CAD build for the part. Positions are in the model's coordinates, mm. Face numbers are marked on the shaded views. A direction names the side the tool comes from. Coordinates: 2 decimals unless noted, no trailing zeros. Order: outer loops, then holes, each group sorted by start corner. A loop starts at its lowest first (then second) coordinate and runs counter-clockwise, first axis right, second up. Notation, with made-up numbers: (2.25, 30) - (21.25, 30) arc R7 ccw to (21.25, 35) - close; hole circle Ø9 at (38.25, -20). An arc over 180 degrees is marked (long way). Return JSON: item names as keys, results as strings.
Autodesk Inventor part; units mm, degrees
ref_plane "XZ Plane" through (0, 0, 0) normal (0, 1, 0) x (-1, 0, 0)
ref_plane "XY Plane" through (0, 0, 0) normal (0, 0, 1) x (1, 0, 0)
sketch "草图1" plane through (0, 0, 0) normal (0, 1, 0) x (-1, 0, 0)
  line L0 (234.2186, 0) -> (-293.6058, 0)
  line L1 (7.25, 23.5) -> (-7.25, 23.5)
  line L2 (-7.25, -23.5) -> (7.25, -23.5)
  line L3 (7.25, -23.5) -> (7.25, 23.5)
  line L4 (7.25, 23.5) -> (-7.25, -23.5) construction
  line L5 (-7.25, 23.5) -> (7.25, -23.5) construction
  line L6 (-7.25, 15.5) -> (-0.75, 15.5)
  line L7 (-0.75, 15.5) -> (-0.75, -15.5)
  line L8 (-0.75, -15.5) -> (-7.25, -15.5)
  line L9 (-13.75, 15.5) -> (-0.75, -15.5) construction
  line L10 (-0.75, 15.5) -> (-13.75, -15.5) construction
  line L11 (-7.25, 23.5) -> (-7.25, 15.5)
  line L12 (-7.25, -15.5) -> (-7.25, -23.5)
  point P0 (0, 0)
  point P1 (-7.25, 0)
  dimension "d0" = 14.5
  dimension "d1" = 47
  dimension "d2" = 13
sketch "草图2" plane through (0, 0, 0) normal (0, 1, 0) x (-1, 0, 0)
  point P0 (0, 0)
sketch "草图3" plane through (0, 0, 0) normal (0, 0, 1) x (1, 0, 0)
  line L0 (0, 0) -> (0, 27)
  arc A0 (32.5, 27) -> (0, 27) centre (16.25, 27) ccw
  line L1 (32.5, 27) -> (32.5, 0)
  dimension "d4" = 27
  dimension "d5" = 32.5
sweep "扫掠1" add profiles "草图1" path "草图3"
sketch "草图4" plane through (7.25, 0, -23.5) normal (0, 0, -1) x (-1, 0, 0)
  line L0 (-18, 27) -> (-18, 0)
  arc A0 (0, 27) -> (-18, 27) centre (-9, 27) ccw
  line L1 (0, 0) -> (0, 27)
  arc A1 (-18, 27) -> (0, 27) centre (-9, 27) ccw
  line L2 (-18, 9) -> (0, 9)
  line L3 (-18, 9) -> (-18, 27)
  line L4 (0, 9) -> (0, 27)
  point P0 (7.25, 0)
  dimension "d7" = 18
extrude "拉伸1" add sketch "草图4" against normal blind 8 contours A1 L1 L2 L0
sketch "草图5" plane through (-7.25, 0, 23.5) normal (0, -1, 0) x (1, 0, 0)
  line L0 (0, 0) -> (14.5, 0)
  line L1 (0, -47) -> (0, 0)
  line L2 (14.5, -47) -> (0, -47)
  line L3 (14.5, -39) -> (14.5, -47)
  line L4 (8, -39) -> (14.5, -39)
  line L5 (8, -8) -> (8, -39)
  line L6 (14.5, -8) -> (8, -8)
  line L7 (14.5, 0) -> (14.5, -8)
  point P0 (7.25, -23.5)
sketch "草图6" plane through (25.25, 0, 23.5) normal (0, -1, 0) x (1, 0, 0)
  line L0 (14.5, 0) -> (0, 0)
  line L1 (0, 0) -> (0, -8)
  line L2 (0, -8) -> (6.5, -8)
  line L3 (6.5, -8) -> (6.5, -39)
  line L4 (6.5, -39) -> (0, -39)
  line L5 (0, -39) -> (0, -47)
  line L6 (0, -47) -> (14.5, -47)
  line L7 (14.5, -47) -> (14.5, 0)
  point P0 (-25.25, -23.5)
sketch "草图7" plane through (-7.25, 0, 23.5) normal (0, -1, 0) x (1, 0, 0)
  line L0 (0, 0) -> (14.5, 0)
  line L1 (0, -47) -> (0, 0)
  line L2 (14.5, -47) -> (0, -47)
  line L3 (14.5, -39) -> (14.5, -47)
  line L4 (8, -39) -> (14.5, -39)
  line L5 (8, -8) -> (8, -39)
  line L6 (14.5, -8) -> (8, -8)
  line L7 (14.5, 0) -> (14.5, -8)
  point P0 (7.25, -23.5)
  dimension "d10" = 6.5
sketch "草图8" plane through (-7.25, 0, 23.5) normal (0, -1, 0) x (1, 0, 0)
  line L0 (8, -8) -> (8, -39)
  circle A0 centre (23.5, -23.5) radius 9
  point P0 (7.25, -23.5)
  dimension "d11" = 18
  dimension "d12" = 15.5
extrude "拉伸2" cut sketch "草图8" against normal blind 232
sketch "草图9" plane through (-7.25, 0, -23.5) normal (-1, 0, 0) x (0, 0, 1)
  line L0 (42.5, 0) -> (4.5, 0)
  line L1 (4.5, 0) -> (4.5, 20)
  line L2 (4.5, 20) -> (42.5, 20)
  line L3 (42.5, 20) -> (42.5, 0)
  line L4 (42.5, 0) -> (4.5, 20) construction
  line L5 (4.5, 0) -> (42.5, 20) construction
  line L6 (47, 0) -> (39, 0)
  point P0 (23.5, 0)
  point P1 (23.5, 10)
  point P2 (43, 0)
  dimension "d15" = 38
  dimension "d16" = 20
ref_plane "工作平面1" through (-3.625, 0, 0) normal (1, 0, 0) x (0, 1, 0)
ref_plane "工作平面2" through (-32.25, 0, -23.5) normal (-1, 0, 0) x (0, 0, 1)
sketch "草图10" plane through (-32.25, 0, -23.5) normal (-1, 0, 0) x (0, 0, 1)
  line L0 (12, 0) -> (35, 0)
  line L1 (35, 0) -> (35, 10)
  line L2 (35, 10) -> (12, 10)
  line L3 (12, 10) -> (12, 0)
  line L4 (12, 0) -> (35, 10) construction
  line L5 (35, 0) -> (12, 10) construction
  point P0 (23.5, 0)
  point P1 (23.5, 5)
  point P2 (39, 0)
  dimension "d18" = 23
  dimension "d19" = 10
loft "放样1" add profiles "草图10", "草图9"
sketch "草图11" plane through (-32.25, 0, 11.5) normal (-1, 0, 0) x (0, 0, 1)
  line L0 (-23, 0) -> (0, 0)
  line L1 (0, 0) -> (0, 10)
  line L2 (0, 10) -> (-23, 10)
  line L3 (-23, 10) -> (-23, 0)
  point P0 (-11.5, 0)
sketch "草图12" plane through (-7.25, 0, 23.5) normal (0, -1, 0) x (1, 0, 0)
  line L0 (-25, -35) -> (-25, -12)
  line L1 (-15, -29.113) -> (-25, -29.113)
  line L2 (-25, -29.113) -> (-25, -17.887)
  line L3 (-25, -17.887) -> (-15, -17.887)
  line L4 (-15, -17.887) -> (-15, -29.113)
  line L5 (-15, -29.113) -> (-25, -17.887) construction
  line L6 (-25, -29.113) -> (-15, -17.887) construction
  point P0 (7.25, -23.5)
  point P1 (-20, -23.5)
  point P2 (-25, -23.5)
  dimension "d24" = 10
extrude "拉伸3" cut sketch "草图12" against normal blind 232
equation "\"折弯半径\" = 厚度"
equation "\"折弯释压宽度\" = 厚度"
equation "\"折弯释压深度\" = 0.5 * 厚度"
equation "\"拐角释压尺寸\" = 4 * 厚度"
equation "\"最小余量\" = 2 * 厚度"
equation "\"过渡半径\" = 折弯半径"
equation "\"Jacobi半径尺寸\" = 厚度"
equation "\"间隙大小\" = 厚度"
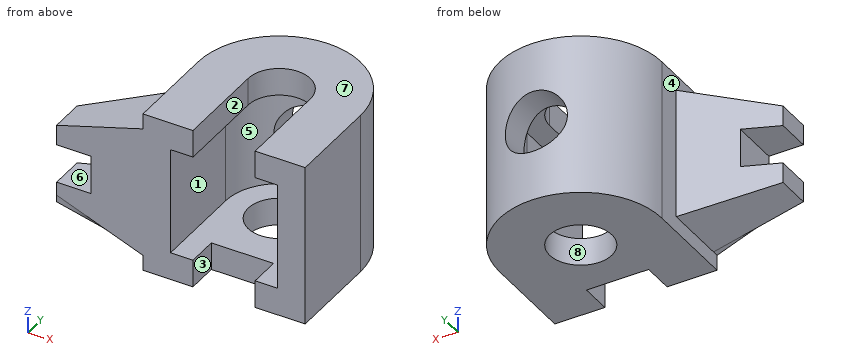
Item 1: Band-saw the part on B-B, the plane y = 38. List the corners of the cut face in (x, z).
Findings below:
{"outline": "(-4.52, -23.5) - (37.02, -23.5) - (37.02, 23.5) - (-4.52, 23.5) - close; hole (5.33, -15.5) - (27.17, -15.5) - (27.17, 15.5) - (5.33, 15.5) - close"}
Item 2: Drop flat-ended pins along their axis: P1, Ø12, axis at x = -14.5, y = 16, coming from the +Z side (3 decimals); P2, Ø8, axis at y = 30, z = 17, coming from the +X side; P3, Ø13.5, axis at y = 20, z = 7, coming from the -X side (3 decimals); P4, Ø3, axis at y = 34, z = -18.5, coming from the -X side. Give the stop position or say it passes through.
Findings below:
{"P1": "stops at z = 18.625", "P2": "stops at x = 39.75", "P3": "stops at x = -24.125", "P4": "stops at x = -6.6"}
Item 3: Wall check: L1, parallel to X at y = 27, z = -20.5; L2, parallel to X at y = 5, z = -2; L3, parallel to Z at x = 16.25, y = 42. Give the ranges that are in metal, low to high. Write a range as [from, to].
Findings below:
{"L1": "x = [-7.25, 7.25], [25.25, 39.75]", "L2": "x = [-22.25, 0.75], [31.75, 39.75]", "L3": "z = [-23.5, -15.5], [15.5, 23.5]"}
Item 4: Mould opens along Z. For the marked faces 5, 6, 7 and 8 say: released by +Z, released by -Z, zero draft, split by the parting line, or undercut.
Findings below:
{"face 5": "undercut", "face 6": "undercut", "face 7": "released by +Z", "face 8": "zero draft"}
Item 5: Which spindle directions (+Z, -Z, +X, -X, +Y, -Y) get a long thin tool onto all of the face, cutting with end or side? Do the marked faces 1, 2, 3 and 4. Say none if no direction does.
Findings below:
{"face 1": "-Y", "face 2": "+Z, -Y", "face 3": "+Z, -Z, -Y", "face 4": "-X, +Y"}
Item 6: Band-saw the part on A-A, the plane x = 16.25. List the corners of the cut face in (y, z).
Findings below:
{"outline": "(9, -23.5) - (18, -23.5) - (18, -15.5) - (9, -15.5) - close; (36, -23.5) - (50.5, -23.5) - (50.5, -9) - (42.5, -9) - (42.5, -15.5) - (36, -15.5) - close; (36, 15.5) - (42.5, 15.5) - (42.5, 9) - (50.5, 9) - (50.5, 23.5) - (36, 23.5) - close"}
Item 7: Band-saw the part on C-C, the plane x = -3.5. List the corners of the cut face in (y, z), then the cut area to 3 significant figures.
Findings below:
{"outline": "(0, -23.5) - (39.74, -23.5) - (39.74, 23.5) - (0, 23.5) - close", "area": "1,870 mm²"}
